```python
from build123d import *

# Parameters (mm, degrees)
SKETCH012_W         = 182
SKETCH012_H         = 160
PAD006_DEPTH        = 20
HOLE005_D           = 7.1
HOLE005_DEPTH       = 25
HOLE005_CBORE_D     = 25
HOLE005_CBORE_DEPTH = 16
SKETCH020_W         = 146
SKETCH020_H         = 125
POCKET004_DEPTH     = 5
POCKET004_TAPER     = 60
CHAMFER001_SIZE     = 2
SKETCH025_W         = 115
SKETCH025_H         = 107
POCKET007_DEPTH     = 12
POCKET014_DEPTH     = 500


with BuildPart() as part:
    # Sketch012 → Pad006 (new body)
    with BuildSketch(Plane.XY):
        with Locations((91, 82)):
            Rectangle(SKETCH012_W, SKETCH012_H)
    extrude(amount=PAD006_DEPTH)

    # Hole005
    with Locations(Plane.XY.offset(20)):
        with Locations((20, 152), (20, 12), (175.5, 147), (175.5, 17)):
            CounterBoreHole(HOLE005_D / 2, HOLE005_CBORE_D / 2, HOLE005_CBORE_DEPTH, depth=HOLE005_DEPTH)

    # Sketch020 → Pocket004 (cut)
    with BuildSketch(Plane.XY):
        with Locations((98, 82.5)):
            Rectangle(SKETCH020_W, SKETCH020_H)
    extrude(amount=POCKET004_DEPTH, taper=POCKET004_TAPER, mode=Mode.SUBTRACT)

    # Chamfer001
    chamfer001_edges = [part.edges().sort_by_distance(p)[0] for p in [
        (104.75, 2, 20),
        (6.25, 2, 20),
        (6.25, 162, 20),
        (104.75, 162, 20),
    ]]
    chamfer(chamfer001_edges, length=CHAMFER001_SIZE)

    # Sketch025 → Pocket007 (cut)
    with BuildSketch(Plane.XY):
        with Locations((91.5, 82.5)):
            Rectangle(SKETCH025_W, SKETCH025_H)
    extrude(amount=POCKET007_DEPTH, mode=Mode.SUBTRACT)

    # Sketch032 → Pocket014 (cut)
    with BuildSketch(Plane.XZ):
        Polygon((140, 30), (190, 30), (190, 10), (170, 10), (160, 10), (158, 10), (140, 22), align=None)
    extrude(amount=-POCKET014_DEPTH, mode=Mode.SUBTRACT)


with BuildPart() as part_1:
    # Body004 placement: moved
    add(part.part.moved(Location((-80, -12, 116))))


solid = part_1.part
```
Work out the finished part from the listing and answer in its coordinate system (mm). A direction names the side the tool comes from. Round coordinates to 2 decimals unless told otherwise and drop trailing zeros. Order: outer loops, then holes, each group sorted by start corner. A loop starts at its lowest first (then second) coordinate and runs counter-clockwise, first axis right, second up.
Q1. A tool of negligible diameter and unlimited length cuts with its end or side. For faces 1 (the flat face through (90, 69, 126)), 2 (the cylindrical face through (-59.563, 12.492, 128.112)), 3 (the flat face through (-46, 70, 124)), 4 (the cylindrical face through (95.96, 138.52, 117.97)), from which of +Z, -Z, +X, -X, +Y, -Y can it reach the whole face along a straight path? Write none if from no direction.
Solution:
face 1: +Z, +X, +Y, -Y
face 2: +Z
face 3: -Z
face 4: +Z, -Z
Q2. Find the intervals of material crossed by line 1 along Y through (x, z) = (-60, 117.75); line 2 along X through (y, z) = (99, 125.75); line 3 along Y through (x, z) = (95.5, 122.3), in increasing order.
Solution:
line 1: y = -10 to -3.55, 3.55 to 136.45, 143.55 to 150
line 2: x = -80 to -46, 69 to 102
line 3: y = -10 to -7.5, 17.5 to 122.5, 147.5 to 150
Q3. A cutting plane is placed at A-A, the plane x = 95.5. Determine the outline of the cut face in (y, z), then the cut area to 3 significant figures.
Solution:
outline: (-10, 116) - (1.45, 116) - (1.45, 120) - (-7.5, 120) - (-7.5, 126) - (-10, 126) - close; (8.55, 116) - (131.45, 116) - (131.45, 120) - (122.5, 120) - (122.5, 126) - (17.5, 126) - (17.5, 120) - (8.55, 120) - close; (138.55, 116) - (150, 116) - (150, 126) - (147.5, 126) - (147.5, 120) - (138.55, 120) - close
area: 1,240 mm2
Q4. The mould has two halves that part along Y. Classify faces 5 (the flat face through (10, 150, 125)), 6 (the flat face through (11, 17, 124)), 7 (the flat face through (10, -10, 125)): pulls with the +Y half, pulls with the -Y half, needs draft (parallel to the pull), parting line crosses it, or undercut.
Solution:
face 5: pulls with the +Y half
face 6: undercut
face 7: pulls with the -Y half
Q5. A cutting plane is placed at C-C, the plane y = 67.5. Determine the outline of the cut face in (x, z), then the cut area to 3 significant figures.
Solution:
outline: (-80, 116) - (-55, 116) - (-46.34, 121) - (-46, 121) - (-46, 128) - (69, 128) - (69, 121) - (82.34, 121) - (91, 116) - (102, 116) - (102, 126) - (78, 126) - (63, 136) - (-80, 136) - close
area: 1,830 mm2
Q6. A cutting plane is placed at D-D, the plane z = 131.5. Determine the outline of the cut face in (x, y), then the cut area to 3 significant figures.
Solution:
outline: (-80, -10) - (-67.5, -10) arc R12.5 cw (long way) to (-52.5, -10) - (69.75, -10) - (69.75, 150) - (-52.5, 150) arc R12.5 cw (long way) to (-67.5, 150) - (-80, 150) - close
area: 23,000 mm2
Q7. Given pin 1 Ø8 at (x, y) = (95.5, 5) entering from +Z; pin 2 Ø12 at (x, y) = (36.5, 77.5) entering from -Z; pin 3 Ø8 at (x, y) = (-60, 0) entering from -Z; pin 4 Ø4 at (x, z) = (-61, 133.5) entering from -Y, each flat-ended and moving along its own axis, determine where each tip first touches the part or whether it passes through.
Solution:
pin 1: stops at z = 120
pin 2: stops at z = 128
pin 3: stops at z = 116
pin 4: stops at y = 12.13
Q8. A cutting plane is placed at B-B, the plane x = 20.5. Determine the outline of the cut face in (y, z).
Solution:
outline: (-10, 116) - (8, 116) - (16.66, 121) - (17, 121) - (17, 128) - (124, 128) - (124, 121) - (124.34, 121) - (133, 116) - (150, 116) - (150, 134) - (148, 136) - (-8, 136) - (-10, 134) - close
